CAD build for the part. Positions are in the model's coordinates, mm. A direction names the side the tool comes from. Round coordinates to 2 decimals unless told otherwise and drop trailing zeros. Write each loop counter-clockwise with the first axis right and the second up, starting at its lowest first coordinate (ties: lowest second). Pieces come first, ordered by that corner, then holes. Notation, with made-up numbers: (18.5, -9.5) - (51.5, -9.5) arc R25 ccw to (51.5, 3.5) - close; hole circle Ø4 at (25.25, -25.5). An arc over 180 degrees is marked (long way). Answer in a Markdown table with one row per item.
```python
from build123d import *

# Parameters (mm, degrees)
SKETCH1_R                      = 6.05
SKETCH1_R_2                    = 3.05
BOSS_EXTRUDE1_DEPTH            = 10
SKETCH2_R                      = 17.5
BOSS_EXTRUDE2_DEPTH            = 6.5
CUT_EXTRUDE1_REACH             = 28.693
SKETCH3_R                      = 1.25
CUT_EXTRUDE2_DEPTH             = 30.744747435
CUT_EXTRUDE2_DEPTH_BACK        = 30.744747435
SKETCH4_R                      = 1.5
CUT_EXTRUDE3_REACH             = 28.693
SKETCH6_R                      = 3.2
CUT_EXTRUDE3_DIRECTION_2_REACH = 28.693
BOSS_EXTRUDE3_DEPTH            = 16.5
SKETCH8_W                      = 5.75
SKETCH8_H                      = 2.75
CUT_EXTRUDE4_DEPTH             = 5
CUT_EXTRUDE5_DEPTH             = 2.75


with BuildPart() as part:
    # Sketch1 → Boss-Extrude1 (new body)
    with BuildSketch(Plane(origin=(0, 0, 0), x_dir=(1, 0, 0), z_dir=(0, 1, 0))):
        with Locations(Location((0, 0, 0), (0, 0, 270))):
            Circle(SKETCH1_R)
        with Locations(Location((0, 0, 0), (0, 0, 270))):
            Circle(SKETCH1_R_2, mode=Mode.SUBTRACT)
    extrude(amount=BOSS_EXTRUDE1_DEPTH)

    # Sketch2 → Boss-Extrude2 (add)
    with BuildSketch(Plane(origin=(0, 10, 0), x_dir=(1, 0, 0), z_dir=(0, 1, 0))):
        with Locations(Location((0, 0, 0), (0, 0, 90))):
            Circle(SKETCH2_R)
    extrude(amount=BOSS_EXTRUDE2_DEPTH)

    # Sketch3 → Cut-Extrude1 (cut, up to next)
    with BuildSketch(Plane.XZ.offset(-10), mode=Mode.PRIVATE) as cut_extrude1_sk1:
        with Locations(Location((12, 0, 0), (0, 0, 270))):
            Circle(SKETCH3_R)
    cut_extrude1_tool1 = extrude(cut_extrude1_sk1.sketch, amount=-CUT_EXTRUDE1_REACH, mode=Mode.PRIVATE) & part.part
    # Sketch3 → Cut-Extrude1 (cut, up to next)
    with BuildSketch(Plane.XZ.offset(-10), mode=Mode.PRIVATE) as cut_extrude1_sk2:
        with Locations(Location((0, -12, 0), (0, 0, 270))):
            Circle(SKETCH3_R)
    cut_extrude1_tool2 = extrude(cut_extrude1_sk2.sketch, amount=-CUT_EXTRUDE1_REACH, mode=Mode.PRIVATE) & part.part
    # Sketch3 → Cut-Extrude1 (cut, up to next)
    with BuildSketch(Plane.XZ.offset(-10), mode=Mode.PRIVATE) as cut_extrude1_sk3:
        with Locations(Location((-12, 0, 0), (0, 0, 270))):
            Circle(SKETCH3_R)
    cut_extrude1_tool3 = extrude(cut_extrude1_sk3.sketch, amount=-CUT_EXTRUDE1_REACH, mode=Mode.PRIVATE) & part.part
    # Sketch3 → Cut-Extrude1 (cut, up to next)
    with BuildSketch(Plane.XZ.offset(-10), mode=Mode.PRIVATE) as cut_extrude1_sk4:
        with Locations(Location((0, 12, 0), (0, 0, 270))):
            Circle(SKETCH3_R)
    cut_extrude1_tool4 = extrude(cut_extrude1_sk4.sketch, amount=-CUT_EXTRUDE1_REACH, mode=Mode.PRIVATE) & part.part
    add(cut_extrude1_tool1.solids().sort_by_distance((12, 10, 0))[0], mode=Mode.SUBTRACT)
    add(cut_extrude1_tool2.solids().sort_by_distance((0, 10, -12))[0], mode=Mode.SUBTRACT)
    add(cut_extrude1_tool3.solids().sort_by_distance((-12, 10, 0))[0], mode=Mode.SUBTRACT)
    add(cut_extrude1_tool4.solids().sort_by_distance((0, 10, 12))[0], mode=Mode.SUBTRACT)

    # Sketch4 → Cut-Extrude2 (cut, two sides: drawn at the far end of the back side and taken through both)
    with BuildSketch(Plane.XY.offset(-CUT_EXTRUDE2_DEPTH_BACK)):
        with Locations((0, 4.916404418)):
            Circle(SKETCH4_R)
    extrude(amount=CUT_EXTRUDE2_DEPTH + CUT_EXTRUDE2_DEPTH_BACK, mode=Mode.SUBTRACT)

    # Sketch6 → Cut-Extrude3 (cut, up to next)
    with BuildSketch(Plane(origin=(0, 10, 0), x_dir=(-1, 0, 0), z_dir=(0, -1, 0)), mode=Mode.PRIVATE) as cut_extrude3_sk1:
        with Locations(Location((0, 0, 0), (0, 0, 270))):
            Circle(SKETCH6_R)
    cut_extrude3_tool1 = extrude(cut_extrude3_sk1.sketch, amount=-CUT_EXTRUDE3_REACH, mode=Mode.PRIVATE) & part.part
    add(cut_extrude3_tool1.solids().sort_by_distance((0, 10, 0))[0], mode=Mode.SUBTRACT)

    # Sketch6 → Cut-Extrude3 direction 2 (cut, up to next)
    with BuildSketch(Plane(origin=(0, 10, 0), x_dir=(-1, 0, 0), z_dir=(0, -1, 0)), mode=Mode.PRIVATE) as cut_extrude3_direction_2_sk1:
        with Locations(Location((0, 0, 0), (0, 0, 270))):
            Circle(SKETCH6_R)
    cut_extrude3_direction_2_tool1 = extrude(cut_extrude3_direction_2_sk1.sketch, amount=CUT_EXTRUDE3_DIRECTION_2_REACH, mode=Mode.PRIVATE) & part.part
    add(cut_extrude3_direction_2_tool1.solids().sort_by_distance((0, 10, 0))[0], mode=Mode.SUBTRACT)

    # Sketch7 → Boss-Extrude3 (add)
    with BuildSketch(Plane.XZ):
        with BuildLine():
            Line((-1.636306817, 2.75), (1.636306817, 2.75))
            ThreePointArc((1.636306817, 2.75), (0, 3.2), (-1.636306817, 2.75))
        make_face()
    extrude(amount=-BOSS_EXTRUDE3_DEPTH)

    # Sketch8 → Cut-Extrude4 (cut)
    with BuildSketch(Plane(origin=(17.5, 0, 0), x_dir=(0, 0, -1), z_dir=(1, 0, 0))):
        with Locations((0, 13.25)):
            Rectangle(SKETCH8_W, SKETCH8_H)
    cut_extrude4 = extrude(amount=-CUT_EXTRUDE4_DEPTH, mode=Mode.SUBTRACT)

    # Sketch9 → Cut-Extrude5 (cut)
    with BuildSketch(Plane.XZ.offset(-14.625)):
        Polygon((15.319764048, 0), (13.659882024, 2.875), (10.340117976, 2.875), (8.680235952, 0), (10.340117976, -2.875), (13.659882024, -2.875), align=None)
    cut_extrude5 = extrude(amount=CUT_EXTRUDE5_DEPTH, mode=Mode.SUBTRACT)

    # Mirror1: Cut-Extrude4, Cut-Extrude5 across plane
    add(cut_extrude4.mirror(Plane(origin=(0, 0, 0), x_dir=(0, 0, 1), z_dir=(1, 0, 0))), mode=Mode.SUBTRACT)
    add(cut_extrude5.mirror(Plane(origin=(0, 0, 0), x_dir=(0, 0, 1), z_dir=(1, 0, 0))), mode=Mode.SUBTRACT)


solid = part.part
```
Q1. Saw through at D-D on x = -12. List the corners of the cut face in (y, z) (3 decimals), then the cut area to 3 significant figures.
Computed:
| item | result |
|---|---|
| outline | (10, -12.738) - (16.5, -12.738) - (16.5, -1.25) - (14.625, -1.25) - (14.625, -2.875) - (11.875, -2.875) - (11.875, -1.25) - (10, -1.25) - close; (10, 1.25) - (11.875, 1.25) - (11.875, 2.875) - (14.625, 2.875) - (14.625, 1.25) - (16.5, 1.25) - (16.5, 12.738) - (10, 12.738) - close |
| area | 140 mm2 |
Q2. Saw through at A-A on x = 0. List the corners of the cut face in (y, z).
Computed:
| item | result |
|---|---|
| outline | (0, -6.05) - (3.42, -6.05) - (3.42, -3.2) - (0, -3.2) - close; (0, 2.75) - (16.5, 2.75) - (16.5, 10.75) - (10, 10.75) - (10, 6.05) - (6.42, 6.05) - (6.42, 3.2) - (3.42, 3.2) - (3.42, 6.05) - (0, 6.05) - close; (6.42, -6.05) - (10, -6.05) - (10, -10.75) - (16.5, -10.75) - (16.5, -3.2) - (6.42, -3.2) - close; (10, -17.5) - (16.5, -17.5) - (16.5, -13.25) - (10, -13.25) - close; (10, 13.25) - (16.5, 13.25) - (16.5, 17.5) - (10, 17.5) - close |
Q3. Saw through at B-B on y = 15.25. List the corners of the cut face in (x, z), then the cut area to 3 significant figures.
Computed:
| item | result |
|---|---|
| outline | circle Ø35 at (0, 0); hole circle Ø2.5 at (-12, 0); hole (-1.64, 2.75) arc R3.2 ccw (long way) to (1.64, 2.75) - close; hole circle Ø2.5 at (0, -12); hole circle Ø2.5 at (0, 12); hole circle Ø2.5 at (12, 0) |
| area | 911 mm2 |
Q4. Drill centre lines: line 1 (X direction, y = 15.8, z = 0); line 2 (Z direction, x = -1, y = 12.5); line 3 (X direction, y = 3.75, z = 0). Where is each one in solid material? Low to high.
Computed:
| item | result |
|---|---|
| line 1 | x = -17.5 to -13.25, -10.75 to -3.2, 3.2 to 10.75, 13.25 to 17.5 |
| line 2 | z = -17.47 to -12.75, -11.25 to -3.04, 2.75 to 11.25, 12.75 to 17.47 |
| line 3 | x = -6.05 to -3.2, 3.2 to 6.05 |
Q5. Flat gauge pins, fed straight in: pin 1 (4 mm diameter, centred on x = 4, y = 4, fed in from +Z); pin 2 (4.5 mm diameter, centred on x = -14, z = -0.5, fed in from -Y); pin 3 (3 mm diameter, centred on x = 3.5, y = 10.5, fed in from +Z). Where does each tip first touch, or does it go through?
Computed:
| item | result |
|---|---|
| pin 1 | stops at z = 5.71 |
| pin 2 | stops at y = 10 |
| pin 3 | stops at z = 17.39 |
Q6. Pull direction X, two halves, no side cores. Call faces 1 (the flat face through (0, 16.5, -4)), 2 (the flat face through (9.5, 13.27, -1.42)), 3 (the cylindrical face through (0.05, 13.2, 13.25)), 4 (the cylindrical face through (1.82, 4.93, 5.77)): released by +X, released by -X, zero draft, split by the parting line, or undercut.
Computed:
| item | result |
|---|---|
| face 1 | zero draft |
| face 2 | released by +X |
| face 3 | undercut |
| face 4 | split by the parting line |
Q7. 3-axis set-ups, long thin cutter, end or side, ignore diameter. For faces 5 (the flat face through (9.522, 13.269, 1.458)), 6 (the flat face through (8, 10, 0)), 7 (the flat face through (-9.522, 13.269, 1.458)), 8 (the cylindrical face through (-10.76, 10.92, 0.16)): which of +Z, -Z, +X, -X, +Y, -Y reach the whole face in a straight line?
Computed:
| item | result |
|---|---|
| face 5 | +X |
| face 6 | -Y |
| face 7 | -X |
| face 8 | +Y, -Y |
Q8. Saw through at C-C on z = 12. List the corners of the cut face in (x, y).
Computed:
| item | result |
|---|---|
| outline | (-12.74, 10) - (-1.25, 10) - (-1.25, 16.5) - (-12.74, 16.5) - close; (1.25, 10) - (12.74, 10) - (12.74, 16.5) - (1.25, 16.5) - close |
